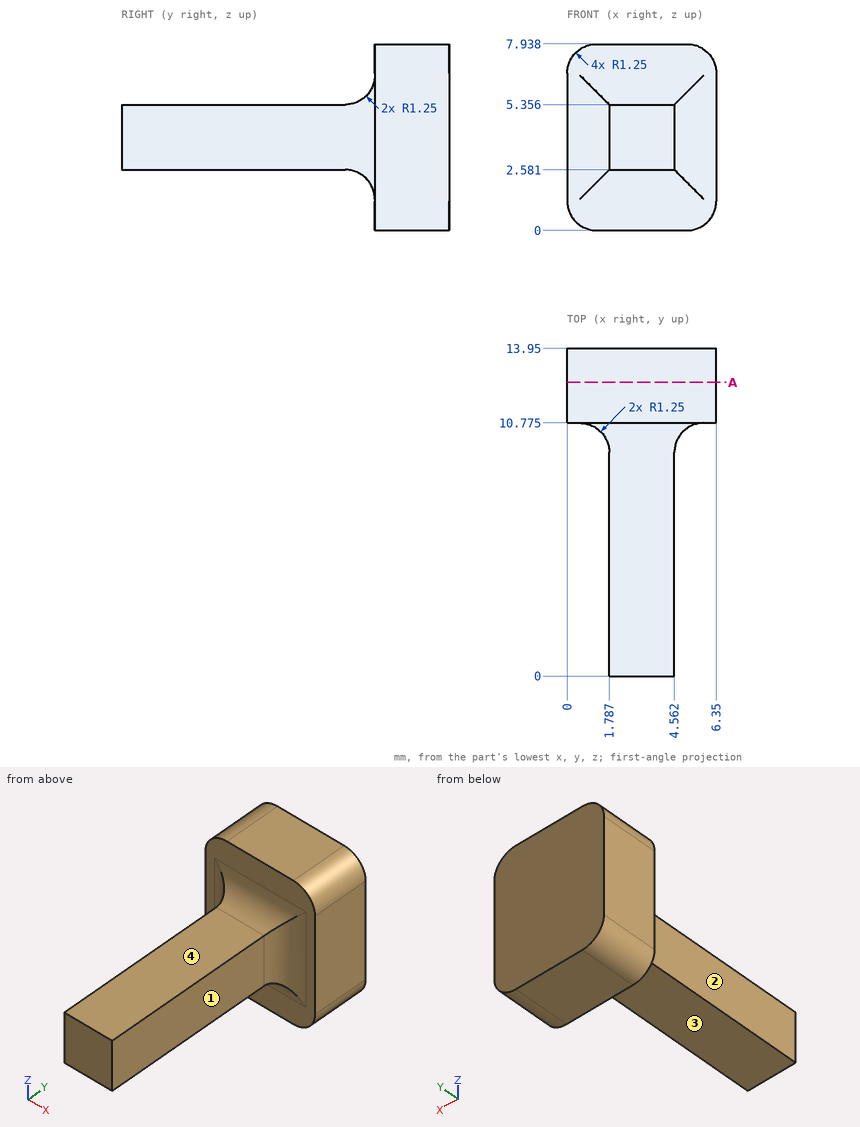
Design review of the part shown in the three views and the two pictorial views. Dimensions are in mm from the part's minimum x, y and z. A direction names the side the tool comes from. Round coordinates to 2 decimals unless told otherwise and drop trailing zeros. Loops run counter-clockwise (first coordinate to the right, second up) from the corner with the lowest first, then second, coordinate; pieces in that order, holes last.
(1) Tool access review of the marked faces 1, 2, 3 and 4: name each direction out of +Z, -Z, +X, -X, +Y, -Y from which nothing blocks a thin tool from reaching the whole face with its end or side.
Returned:
face 1: +Z, -Z, +X, -Y
face 2: +Z, -Z, -X, -Y
face 3: -Z, +X, -X, -Y
face 4: +Z, +X, -X, -Y
(2) Clearance check with flat-ended pins moving along their axes: P1, Ø4, axis at y = 6, z = 3.5, coming from the -X side; P2, Ø1.5, axis at x = 5.5, z = 7, coming from the -Y side; P3, Ø2, axis at x = 3, y = 3.5, coming from the +Z side. State where each tip first meets the part, or that it passes through.
Returned:
P1: stops at x = 1.79
P2: stops at y = 10.72
P3: stops at z = 5.36
(3) We need section A-A (y = 12.5). Give the boundary of the cut face in (x, z).
Returned:
outline: (0, 1.25) arc R1.25 ccw to (1.25, 0) - (5.1, 0) arc R1.25 ccw to (6.35, 1.25) - (6.35, 6.69) arc R1.25 ccw to (5.1, 7.94) - (1.25, 7.94) arc R1.25 ccw to (0, 6.69) - close
(4) Wall thickness on line 1 along Z through (x, y) = (4.5, 4); line 2 along X through (y, z) = (5, 5); line 3 along Y through (x, z) = (3.5, 1.5): over which ranges is each line inside the solid? List them lowest first.
Returned:
line 1: z = 2.58 to 5.36
line 2: x = 1.79 to 4.56
line 3: y = 10.76 to 13.95
